Design review of the part built by this model. Coordinates are the model's own, in mm. Face numbers are marked on the shaded views. A direction names the side the tool comes from. Give positions to 0.01 mm unless a question says otherwise; leave off trailing zeros. Order: outer loops, then holes, each group sorted by start corner. A loop starts at its lowest first (then second) coordinate and runs counter-clockwise, first axis right, second up. Notation, with made-up numbers: (17, 60) -> (60, 60) arc R26 ccw to (60, 95) -> close; hole circle Ø9 at (-5, 39.25). An arc over 180 degrees is marked (long way). Return JSON: item names as keys, results as strings.
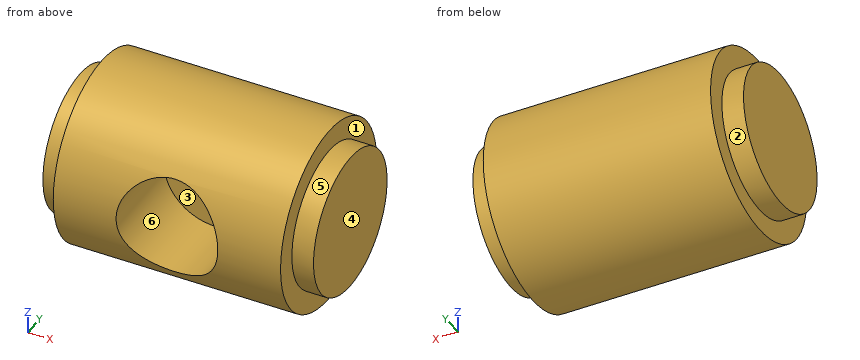
```python
from build123d import *

# Parameters (mm, degrees)
ENL_V_MAT_EXTRU_1_REACH = 10.5
ESQUISSE2_R             = 4.7


with BuildPart() as part:
    # Esquisse1 → Révolution1 (revolve)
    with BuildSketch(Plane.XY, mode=Mode.PRIVATE) as r_volution1_sk:
        Polygon((-25, 0), (0, 0), (0, -6.5), (-2, -6.5), (-2, -8.5), (-23, -8.5), (-23, -6.5), (-25, -6.5), align=None)
    revolve(r_volution1_sk.sketch.rotate(Axis((35.066018426, 0, 0), (-1, 0, 0)), 270), axis=Axis((35.066018426, 0, 0), (-1, 0, 0)))  # turned: the seam where the file's is

    # Esquisse2 → Enlèv. mat.-Extru.1 (cut, up to next)
    with BuildSketch(Plane(origin=(0, 0, 0), x_dir=(1, 0, 0), z_dir=(0, 1, 0)), mode=Mode.PRIVATE) as enl_v_mat_extru_1_sk1:
        with Locations(Location((-12.5, 0, 0), (0, 0, 270))):  # turned: the seam where the file's is
            Circle(ESQUISSE2_R)
    enl_v_mat_extru_1_tool1 = extrude(enl_v_mat_extru_1_sk1.sketch, amount=-ENL_V_MAT_EXTRU_1_REACH, mode=Mode.PRIVATE) & part.part
    add(enl_v_mat_extru_1_tool1.solids().sort_by_distance((-12.5, 0, 0))[0], mode=Mode.SUBTRACT)


solid = part.part
```
Item 1: Machinability: for the marked faces 1, 2 and 3, which of the approach directions +Z, -Z, +X, -X, +Y, -Y give a long, thin tool a straight path to every point of the face, cutting with its end or side? Answer none if there is none.
Result set:
{"face 1": "+X", "face 2": "-X", "face 3": "-Y"}
Item 2: Add section A-A (z = 0). Give the boundary of the cut face in (x, y).
Result set:
{"outline": "(-25, -6.5) -> (-23, -6.5) -> (-23, -8.5) -> (-17.2, -8.5) -> (-17.2, 0) -> (-7.8, 0) -> (-7.8, -8.5) -> (-2, -8.5) -> (-2, -6.5) -> (0, -6.5) -> (0, 6.5) -> (-2, 6.5) -> (-2, 8.5) -> (-23, 8.5) -> (-23, 6.5) -> (-25, 6.5) -> close"}
Item 3: Add section B-B (y = -1). Give the boundary of the cut face in (x, z).
Result set:
{"outline": "(-25, -6.42) -> (-23, -6.42) -> (-23, -8.44) -> (-2, -8.44) -> (-2, -6.42) -> (0, -6.42) -> (0, 6.42) -> (-2, 6.42) -> (-2, 8.44) -> (-23, 8.44) -> (-23, 6.42) -> (-25, 6.42) -> close; hole circle Ø9.4 at (-12.5, 0)"}
Item 4: Add section D-D (y = 2.75). Give the boundary of the cut face in (x, z).
Result set:
{"outline": "(-25, -5.89) -> (-23, -5.89) -> (-23, -8.04) -> (-2, -8.04) -> (-2, -5.89) -> (0, -5.89) -> (0, 5.89) -> (-2, 5.89) -> (-2, 8.04) -> (-23, 8.04) -> (-23, 5.89) -> (-25, 5.89) -> close"}
Item 5: Mouldability with a two-part tool opening along Z and no side actions: class the marked faces 4, 5 and 6 as released by +Z, released by -Z, zero draft, split by the parting line, or undercut.
Result set:
{"face 4": "zero draft", "face 5": "split by the parting line", "face 6": "undercut"}
Item 6: For pin 1 (10 mm diameter, centred on x = -4.5, z = -5, fed in from -Y); pin 2 (5 mm diameter, centred on x = -20, z = 3.5, fed in from -Y); pin 3 (3 mm diameter, centred on x = -16, y = -4.5, fed in from +Z); pin 4 (8 mm diameter, centred on x = -12, y = -6.5, fed in from +Z), all flat-tipped, find the tip position at first contact; note any pin that passes through.
Result set:
{"pin 1": "stops at y = -8.5", "pin 2": "stops at y = -8.44", "pin 3": "stops at z = 7.95", "pin 4": "stops at z = 8.12"}
Item 7: Add section C-C (x = -18). Give the boundary of the cut face in (y, z).
Result set:
{"outline": "circle Ø17 at (0, 0)"}
Item 8: Wall thickness on L1, parallel to X at y = -2.75, z = 0; L2, parallel to X at y = -5.5, z = -1.5; L3, parallel to Z at x = -12.5, y = -3.25: over which ranges is each line inside the solid? List them lowest first. Write a range as [from, to].
Result set:
{"L1": "x = [-25, -17.2], [-7.8, 0]", "L2": "x = [-25, -16.95], [-8.05, 0]", "L3": "z = [-7.85, -4.7], [4.7, 7.85]"}
